Design review of the part built by this model. Coordinates are the model's own, in mm. Coordinates: 2 decimals unless noted, no trailing zeros. Loops run counter-clockwise (first coordinate to the right, second up) from the corner with the lowest first, then second, coordinate; pieces in that order, holes last. Notation, with made-up numbers: (70, 77.5) -> (88, 77.5) arc R14 ccw to (88, 87.5) -> close; hole circle Ø10 at (86.5, -13). An arc over 180 degrees is marked (long way). Use one line per item in the form item = value. Start each with the question number.
1. For pin 1 (3 mm diameter, centred on x = 10, z = -30, fed in from -Y), flat-tipped, find the tip position at first contact; note if it passes through.
2. Wall thickness on line 1 (Z direction, x = 205, y = 13.25); line 2 (X direction, y = 6.25, z = -112); line 3 (X direction, y = 14, z = -470): over which ranges is each line inside the solid? List them lowest first. Write a range as from..to.
3. Consider section B-B (y = 9). State how many separate pieces and enclosed holes the cut face has, then the cut area to 3 significant figures.
4. Consider section A-A (z = -240). State the section outline as (x, y) points, then the cut area to 3 significant figures.
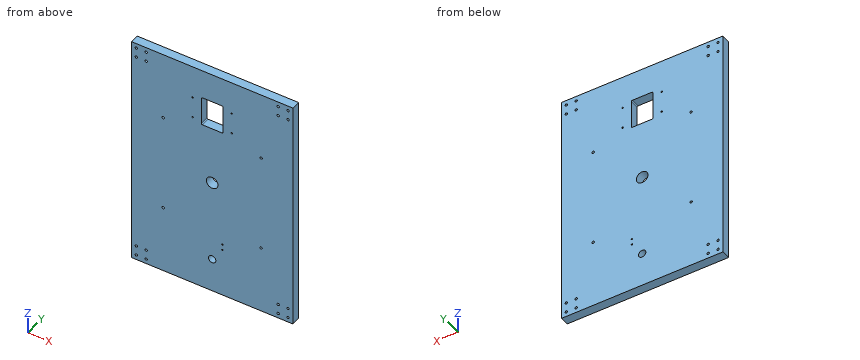
from build123d import *

# Parameters (mm, degrees)
SKETCH1_W           = 330
SKETCH1_H           = 480
SKETCH1_R           = 2.5
SKETCH1_R_2         = 12
SKETCH1_R_3         = 1.5
SKETCH1_R_4         = 7.5
BOSS_EXTRUDE1_DEPTH = 18


with BuildPart() as part:
    # Sketch1 → Boss-Extrude1 (new body)
    with BuildSketch(Plane(origin=(0, 0, 0), x_dir=(1, 0, 0), z_dir=(0, 1, 0))):
        with Locations((165, 240)):
            Rectangle(SKETCH1_W, SKETCH1_H)
        with Locations((10, 10)):
            Circle(SKETCH1_R, mode=Mode.SUBTRACT)
        with Locations((30, 10)):
            Circle(SKETCH1_R, mode=Mode.SUBTRACT)
        with Locations((10, 30)):
            Circle(SKETCH1_R, mode=Mode.SUBTRACT)
        with Locations((30, 30)):
            Circle(SKETCH1_R, mode=Mode.SUBTRACT)
        with Locations((320, 30)):
            Circle(SKETCH1_R, mode=Mode.SUBTRACT)
        with Locations((320, 10)):
            Circle(SKETCH1_R, mode=Mode.SUBTRACT)
        with Locations((300, 10)):
            Circle(SKETCH1_R, mode=Mode.SUBTRACT)
        with Locations((300, 30)):
            Circle(SKETCH1_R, mode=Mode.SUBTRACT)
        with Locations((300, 470)):
            Circle(SKETCH1_R, mode=Mode.SUBTRACT)
        with Locations((320, 470)):
            Circle(SKETCH1_R, mode=Mode.SUBTRACT)
        with Locations((320, 450)):
            Circle(SKETCH1_R, mode=Mode.SUBTRACT)
        with Locations((300, 450)):
            Circle(SKETCH1_R, mode=Mode.SUBTRACT)
        with Locations((30, 470)):
            Circle(SKETCH1_R, mode=Mode.SUBTRACT)
        with Locations((10, 470)):
            Circle(SKETCH1_R, mode=Mode.SUBTRACT)
        with Locations((10, 450)):
            Circle(SKETCH1_R, mode=Mode.SUBTRACT)
        with Locations((30, 450)):
            Circle(SKETCH1_R, mode=Mode.SUBTRACT)
        with Locations((65, 140)):
            Circle(SKETCH1_R, mode=Mode.SUBTRACT)
        with Locations((65, 340)):
            Circle(SKETCH1_R, mode=Mode.SUBTRACT)
        with Locations((265, 140)):
            Circle(SKETCH1_R, mode=Mode.SUBTRACT)
        with Locations((265, 340)):
            Circle(SKETCH1_R, mode=Mode.SUBTRACT)
        with Locations((165, 240)):
            Circle(SKETCH1_R_2, mode=Mode.SUBTRACT)
        with Locations((125, 112)):
            Circle(SKETCH1_R_3, mode=Mode.SUBTRACT)
        with Locations((125, 68)):
            Circle(SKETCH1_R_3, mode=Mode.SUBTRACT)
        with Locations((205, 112)):
            Circle(SKETCH1_R_3, mode=Mode.SUBTRACT)
        with Locations((205, 68)):
            Circle(SKETCH1_R_3, mode=Mode.SUBTRACT)
        with Locations((186, 368)):
            Circle(SKETCH1_R_3, mode=Mode.SUBTRACT)
        with Locations((186, 380)):
            Circle(SKETCH1_R_3, mode=Mode.SUBTRACT)
        with Locations((165, 410)):
            Circle(SKETCH1_R_4, mode=Mode.SUBTRACT)
        with BuildLine():
            Line((145, 60), (185, 60))
            ThreePointArc((185, 60), (186.414213562, 60.585786438), (187, 62))
            Line((187, 62), (187, 118))
            ThreePointArc((187, 118), (186.414213562, 119.414213562), (185, 120))
            Line((185, 120), (145, 120))
            ThreePointArc((145, 120), (143.585786438, 119.414213562), (143, 118))
            Line((143, 118), (143, 62))
            ThreePointArc((143, 62), (143.585786438, 60.585786438), (145, 60))
        make_face(mode=Mode.SUBTRACT)
    extrude(amount=BOSS_EXTRUDE1_DEPTH)


solid = part.part
Geometry check:
q1.pin_1 = through
q2.line_1 = -480..-113.5, -110.5..-69.5, -66.5..0
q2.line_2 = 0..123.5, 126.5..143, 187..203.5, 206.5..330
q2.line_3 = 0..7.5, 12.5..27.5, 32.5..297.5, 302.5..317.5, 322.5..330
q3.separate_pieces = 1
q3.enclosed_holes = 29
q3.area = 155,000 mm²
q4.outline = (0, 0) -> (153, 0) -> (153, 18) -> (0, 18) -> close; (177, 0) -> (330, 0) -> (330, 18) -> (177, 18) -> close
q4.area = 5,510 mm²
